Geometry: final body of the model. Coordinates: model frame, mm. A direction names the side the tool comes from. Round coordinates to 2 decimals unless told otherwise and drop trailing zeros. Write each loop counter-clockwise with the first axis right and the second up, starting at its lowest first coordinate (ties: lowest second). Pieces come first, ordered by that corner, then holes. Notation, with made-up numbers: (80.5, 2) - (124.5, 2) arc R26 ccw to (124.5, 33) - close; hole circle Ø6 at (59.25, -32.5). An arc over 180 degrees is marked (long way). Use a Markdown table: item, result. Add a question column.
```python
from build123d import *

# Parameters (mm, degrees)
F3_W     = 17.1
F3_H     = 36
F0_DEPTH = 5.5
F4_W     = 30
F4_H     = 3
F1_DEPTH = 5.5
F2_SIZE  = 2.99999


# Not quite as in the source:
# - a fillet or chamfer is up to 0.001 mm smaller than in the source, because OpenCascade refuses the exact size


with BuildPart() as f0:
    # F3 (on Top) → F0 (new body, symmetric)
    with BuildSketch(Plane.XY):
        Rectangle(F3_W, F3_H)
    extrude(amount=F0_DEPTH, both=True)

    # F4 (on Right) → F1 (cut, symmetric)
    with BuildSketch(Plane.YZ):
        with Locations((0, 4)):
            Rectangle(F4_W, F4_H)
    extrude(amount=F1_DEPTH, both=True, mode=Mode.SUBTRACT)

    # F2 (size 3 in the source; OpenCascade refuses exactly that, so slightly less here)
    f2_edges = [f0.edges().sort_by_distance(p)[0] for p in [
        (-5.5, 0, 2.5),
        (0, -15, 2.5),
        (0, 15, 2.5),
        (5.5, 0, 2.5),
    ]]
    chamfer(f2_edges, length=F2_SIZE)


solid = f0.part
```
1) Set-up query: faces 5 (the flat face through (-0.1, 13.8, 4.3)), 6 (the flat face through (0, 18, 0)). Return all of +Z, -Z, +X, -X, +Y, -Y with unobstructed straight access to the full face (end or side cutting, diameter ignored); none if empty.
2) Section B-B, the plane z = 3.75. Return the cut outline in (x, y), then the cut area to 3 significant figures.
3) Material intervals for L1, parallel to Z at x = 0.5, y = 10; L2, parallel to Y at x = -2.75, z = 3.5; L3, parallel to X at y = 0, z = 4.5, sorted ascending. Write a range as from..to.
4) Draft query along X for faces 1 (the flat face through (8.55, 0, 0)), 2 (the flat face through (0, 0, 2.5)), 3 (the flat face through (-8.55, 0, 0)), 4 (the flat face through (0, -18, 0)). Return one class per face: released by +X, released by -X, zero draft, split by the parting line, or undercut.
5) Pin query (flat end, axial travel): P1, Ø4, axis at x = 1, y = -4, coming from the +Z side. Return the tip coordinate at first contact, or that it passes through.
Output values:
| question | item | result |
|---|---|---|
| 1 | face 5 | +Z |
| 1 | face 6 | +Z, -Z, +X, -X, +Y |
| 2 | outline | (-8.55, -18) - (8.55, -18) - (8.55, 18) - (-8.55, 18) - close; hole (-3.75, -13.25) - (3.75, -13.25) - (3.75, 13.25) - (-3.75, 13.25) - close |
| 2 | area | 417 mm^2 |
| 3 | L1 | z = -5.5..2.5 |
| 3 | L2 | y = -18..-13, 13..18 |
| 3 | L3 | x = -8.55..-4.5, 4.5..8.55 |
| 4 | face 1 | released by +X |
| 4 | face 2 | undercut |
| 4 | face 3 | released by -X |
| 4 | face 4 | zero draft |
| 5 | P1 | stops at z = 3 |
